Geometry: final body of the model. Coordinates: model frame, mm. Face numbers are marked on the shaded views. Round coordinates to 2 decimals unless told otherwise and drop trailing zeros. Order: outer loops, then holes, each group sorted by start corner. A loop starts at its lowest first (then second) coordinate and runs counter-clockwise, first axis right, second up. Notation, with made-up numbers: M 32,10 L 66,10 A31 ccw 66,34 Z; hole C 23.25,36.25 d6. An arc over 180 degrees is marked long. Put each result on its own line as item: value. Start each with the question number.
1) Section D-D, the plane x = 14.5. Return loops of the section in (y, z), then the cut area to 3 significant figures.
2) Section B-B, the plane z = 90. Return loops of the section in (x, y).
3) Draft query along X for the marked faces 1, 2 and 3. Return one class per face: pulls with the +X half, pulls with the -X half, needs draft (parallel to the pull), parting line crosses it, or undercut.
4) Section C-C, the plane z = 69. Return loops of the section in (x, y), then the cut area to 3 significant figures.
5) First-contact query: P1, Ø4.5, axis at y = -2.24, z = 90, coming from the +X side; P2, Ø10, axis at x = 14.5, z = 97.5, coming from the +Y side. Flat tips, straight axial feed; report the tip coordinate or a pass-through.
6) Material intervals for probe 1 along X at (y, z) = (-3.5, 63); probe 2 along Y at (x, z) = (44, 90); probe 3 along Y at (x, z) = (23, 105), sorted ascending. Write a range as [from, to].
7) Section A-A, the plane y = -6.5. Return loops of the section in (x, z), then the cut area to 3 significant figures.
from build123d import *

# Parameters (mm, degrees)
SKIZZE1_W                            = 50
SKIZZE1_H                            = 20
AUFSATZ_LINEAR_AUSTRAGEN1_DEPTH      = 200
SKIZZE3_R                            = 2.5
SCHNITT_LINEAR_AUSTRAGEN1_DEPTH      = 46.342127859
SCHNITT_LINEAR_AUSTRAGEN1_DEPTH_BACK = 5.657872141
SCHNITT_LINEAR_START                 = 10
SKIZZE4_W                            = 40
SKIZZE4_H                            = 200
SCHNITT_LINEAR_AUSTRAGEN2_DEPTH      = 20


with BuildPart() as part:
    # Skizze1 → Aufsatz-Linear austragen1 (new body)
    with BuildSketch(Plane.XY):
        with Locations((20.342127859, -5.74485208)):
            Rectangle(SKIZZE1_W, SKIZZE1_H)
    extrude(amount=AUFSATZ_LINEAR_AUSTRAGEN1_DEPTH)

    # Skizze3 → Schnitt-Linear austragen1 (cut, two sides)
    with BuildSketch(Plane(origin=(0, 0, 0), x_dir=(0, 0, -1), z_dir=(1, 0, 0))) as schnitt_linear_austragen1_sk:
        with Locations((-90, -2.24485208)):
            Circle(SKIZZE3_R)
        with Locations((-110, -2.24485208)):
            Circle(SKIZZE3_R)
    extrude(amount=SCHNITT_LINEAR_AUSTRAGEN1_DEPTH, mode=Mode.SUBTRACT)
    extrude(schnitt_linear_austragen1_sk.sketch, amount=-SCHNITT_LINEAR_AUSTRAGEN1_DEPTH_BACK, mode=Mode.SUBTRACT)

    # Skizze4 → Schnitt-Linear austragen2 (cut)
    with BuildSketch(Plane(origin=(0, 0, 0), x_dir=(1, 0, 0), z_dir=(0, 1, 0)).offset(SCHNITT_LINEAR_START)):
        with Locations((20.342127859, -100)):
            Rectangle(SKIZZE4_W, SKIZZE4_H)
    extrude(amount=-SCHNITT_LINEAR_AUSTRAGEN2_DEPTH, mode=Mode.SUBTRACT)


solid = part.part
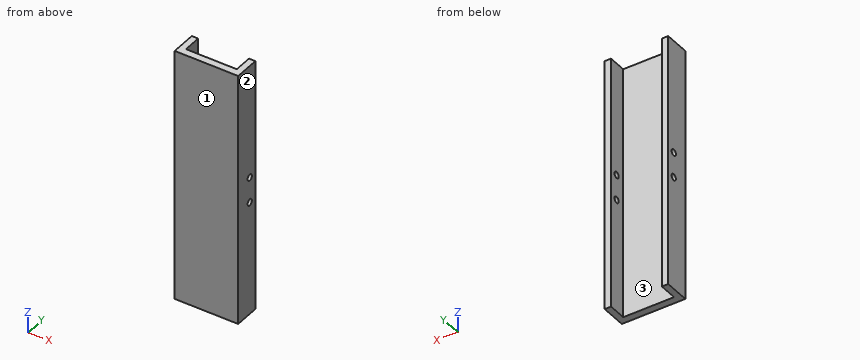
Result sheet:
1. outline: M -15.74,0 L -10,0 L -10,200 L -15.74,200 Z
1. area: 1,150 mm2
2. outline: M -4.66,-15.74 L 45.34,-15.74 L 45.34,-4.74 L 40.34,-4.74 L 40.34,-10 L 0.34,-10 L 0.34,-4.74 L -4.66,-4.74 Z; M -4.66,0.26 L 0.34,0.26 L 0.34,4.26 L -4.66,4.26 Z; M 40.34,0.26 L 45.34,0.26 L 45.34,4.26 L 40.34,4.26 Z
3. face 1: needs draft
3. face 2: pulls with the +X half
3. face 3: undercut
4. outline: M -4.66,-15.74 L 45.34,-15.74 L 45.34,4.26 L 40.34,4.26 L 40.34,-10 L 0.34,-10 L 0.34,4.26 L -4.66,4.26 Z
4. area: 430 mm2
5. P1: passes through
5. P2: stops at y = -10
6. probe 1: x = [-4.66, 0.34], [40.34, 45.34]
6. probe 2: y = [-15.74, -4.74], [0.26, 4.26]
6. probe 3: y = [-15.74, -10]
7. outline: M -4.66,0 L 0.34,0 L 0.34,200 L -4.66,200 Z; M 40.34,0 L 45.34,0 L 45.34,200 L 40.34,200 Z
7. area: 2,000 mm2
